The figure shows three views and two pictorial views of one solid part (mm, origin at its lowest corner). Answer the questions. Give positions to 0.01 mm unless a question says otherwise; leave off trailing zeros. Order: outer loops, then holes, each group sorted by start corner. A loop starts at its lowest first (then second) coordinate and runs counter-clockwise, first axis right, second up. Notation, with made-up numbers: (62, 72) -> (75, 72) arc R30 cw to (75, 107) -> close; hole circle Ø1 at (82.5, 48). An arc over 180 degrees is marked (long way). One line per item, written item: value. Start each with the question number.
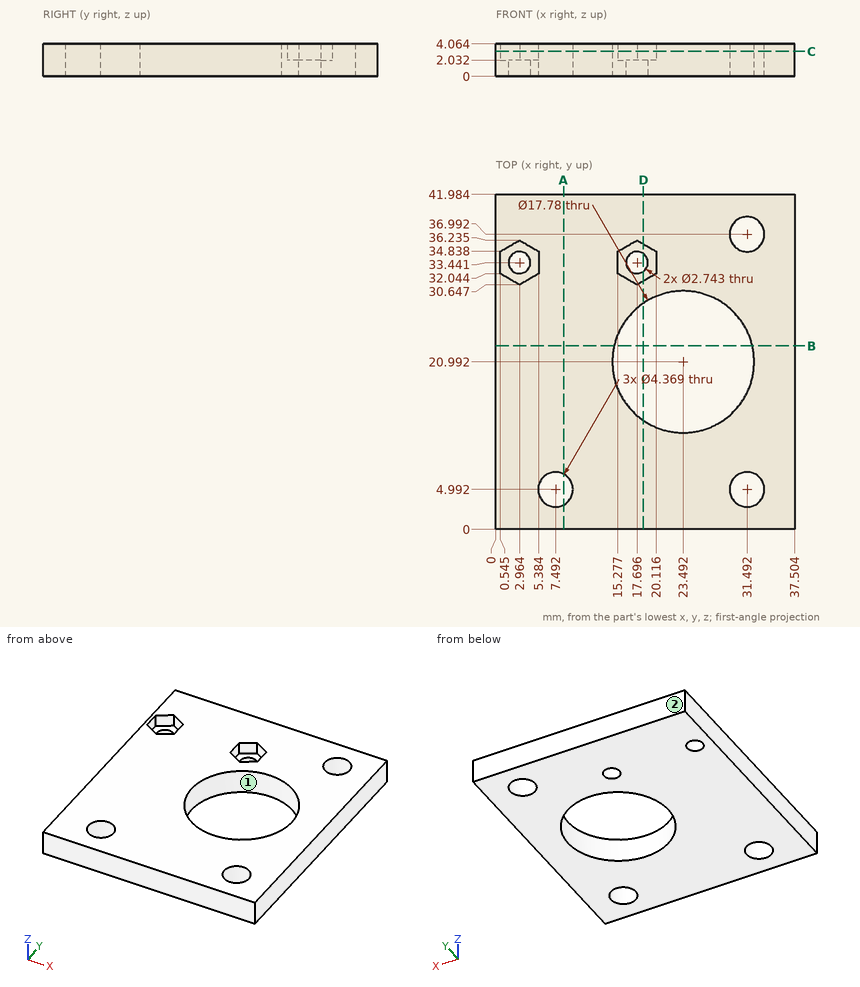
Item 1: Find section C-C on z = 3.15. Write down the section's boundary in (x, y) (1 decimal).
Item 2: Flat-ended cylindrical pins translate along their axes: pin 1 (2.5 mm diameter, centred on x = 7.492, y = 4.992, fed in from +Z); pin 2 (4 mm diameter, centred on x = 2, y = 34.5, fed in from +Z). Find the tip coordinate at first contact, or state that the pin passes through.
Item 3: Find section B-B on y = 23. Write down the section's boundary in (x, z) (1 decimal).
Item 4: Find section D-D on x = 18.5. Write down the section's boundary in (y, z) (1 decimal).
Item 5: Find section A-A on x = 8.5. Write down the section's boundary in (y, z) (1 decimal).
Item 6: For a pull along X with two mould halves and no side action, classify the marked faces 1 and 2 as +X half, -X half, draft (parallel to the pull), parting line (faces both ways), or undercut.
Item 7: Find the intervals of material crossed by line 1 (Y direction, x = 33, z = 0.8) (1 decimal); line 2 (Y direction, x = 23, z = 1.1) (1 decimal); line 3 (Y direction, x = 18, z = 1.7) (1 decimal), in increasing order. Write a range as from..to.
Checks:
1. outline: (0, 0) -> (37.5, 0) -> (37.5, 42) -> (0, 42) -> close; hole (0.5, 32) -> (3, 30.6) -> (5.4, 32) -> (5.4, 34.8) -> (3, 36.2) -> (0.5, 34.8) -> close; hole circle Ø4.4 at (7.5, 5); hole circle Ø17.8 at (23.5, 21); hole (15.3, 32) -> (17.7, 30.6) -> (20.1, 32) -> (20.1, 34.8) -> (17.7, 36.2) -> (15.3, 34.8) -> close; hole circle Ø4.4 at (31.5, 5); hole circle Ø4.4 at (31.5, 37)
2. pin 1: through
2. pin 2: z = 4.06
3. outline: (0, 0) -> (14.8, 0) -> (14.8, 4.1) -> (0, 4.1) -> close; (32.2, 0) -> (37.5, 0) -> (37.5, 4.1) -> (32.2, 4.1) -> close
4. outline: (0, 0) -> (13.6, 0) -> (13.6, 4.1) -> (0, 4.1) -> close; (28.3, 0) -> (32.3, 0) -> (32.3, 2) -> (31.1, 2) -> (31.1, 4.1) -> (28.3, 4.1) -> close; (34.6, 0) -> (42, 0) -> (42, 4.1) -> (35.8, 4.1) -> (35.8, 2) -> (34.6, 2) -> close
5. outline: (0, 0) -> (3.1, 0) -> (3.1, 4.1) -> (0, 4.1) -> close; (6.9, 0) -> (42, 0) -> (42, 4.1) -> (6.9, 4.1) -> close
6. face 1: undercut
6. face 2: draft
7. line 1: 0..3.4, 6.6..35.4, 38.6..42
7. line 2: 0..12.1, 29.9..42
7. line 3: 0..14, 28..32.1, 34.8..42
